Read the model definition and answer for the solid it produces. Units are mm, in the model's axes. A direction names the side the tool comes from. Give positions to 0.01 mm unless a question says otherwise; leave off trailing zeros. Order: outer loops, then holes, each group sorted by start corner. A loop starts at its lowest first (then second) coordinate and runs counter-clockwise, first axis right, second up. Notation, with made-up numbers: (72, 81) - (104, 81) arc R19 ccw to (104, 111) - close; hole circle Ø7 at (-25, 81.5). An arc over 180 degrees is marked (long way). Use a Markdown table: item, result. Add a question column.
1. Which of the six approach directions +Z, -Z, +X, -X, +Y, -Y give full straight-line access (tool end or side, diameter ignored) to faces 5 (the flat face through (11.112, 20, 1)), 6 (the cylindrical face through (0.22, 9.65, 1.48))?
2. A cutting plane is placed at C-C on y = 61.5. Determine the outline of the cut face in (x, z), and give its area (3 significant figures).
3. A cutting plane is placed at B-B on z = 2.3. Determine the outline of the cut face in (x, y) (1 decimal), and give its area (3 significant figures).
4. Flat-ended cylindrical pins translate along their axes: P1, Ø5.5, axis at x = 0, y = -7.94, coming from the -Z side; P2, Ø1.5, axis at y = 11, z = 2, coming from the +X side. Find the tip coordinate at first contact, or state that the pin passes through.
5. A cutting plane is placed at A-A on x = 0. Determine the outline of the cut face in (y, z), and give its area (3 significant figures).
6. A cutting plane is placed at D-D on x = 17.5. Determine the outline of the cut face in (y, z), and give its area (3 significant figures).
7. For a pull along X with two mould halves and no side action, classify faces 1 (the flat face through (4, 46, 3)), 2 (the cylindrical face through (-0.22, -11.11, 1.48)), 3 (the cylindrical face through (0.225, -6.225, 1.479)), 4 (the cylindrical face through (-6.212, 0.076, 1.479)) as released by +X, released by -X, zero draft, split by the parting line, or undercut.
8. Consider L1, parallel to Y at x = 21.5, z = 2.4; L2, parallel to X at y = 24, z = 0.85; L3, parallel to X at y = 88.5, z = 2. Determine where each line is inside the solid, lowest interval first.
```python
from build123d import *

# Parameters (mm, degrees)
BOSS_EXTRU_3_DEPTH   = 3
D_GAGEMENT_51_D      = 3.4544
D_GAGEMENT_M71_D     = 7.6
D_GAGEMENT_M71_DEPTH = 7.01
D_GAGEMENT_M71_TIP   = 2.283270352


with BuildPart() as part:
    # Esquisse1 → Boss.-Extru.3 (new body)
    with BuildSketch(Plane.XY):
        with BuildLine():
            Line((11.1125, 0), (11.1125, 40))
            ThreePointArc((11.1125, 40), (15.168988239, 68.192952149), (27.009351017, 94.098616722))
            ThreePointArc((27.009351017, 94.098616722), (25.537478416, 100.990911223), (18.635346271, 99.565883395))
            ThreePointArc((18.635346271, 99.565883395), (-3.639418742, 51.966145876), (-11.112370677, -0.053611501))
            ThreePointArc((-11.112370677, -0.053611501), (0.026805829, -11.112467669), (11.1125, 0))
        make_face()
    extrude(amount=BOSS_EXTRU_3_DEPTH)

    # Dégagement #51 (through all)
    with Locations(Plane.XY.offset(3)):
        with Locations((-7.9375, 0), (0, 7.9375), (7.9375, 0), (0, -7.9375)):
            Hole(D_GAGEMENT_51_D / 2)

    # Dégagement M71
    with Locations(Plane.XY.offset(3)):
        with Locations((0, 0)):
            Hole(D_GAGEMENT_M71_D / 2, depth=D_GAGEMENT_M71_DEPTH)
            with Locations((0, 0, -(D_GAGEMENT_M71_DEPTH + D_GAGEMENT_M71_TIP / 2))):  # 118° drill point
                Cone(0, D_GAGEMENT_M71_D / 2, D_GAGEMENT_M71_TIP, mode=Mode.SUBTRACT)


solid = part.part
```
Output values:
| question | item | result |
|---|---|---|
| 1 | face 5 | +Z, -Z, +X, -Y |
| 1 | face 6 | +Z, -Z |
| 2 | outline | (-0.5, 0) - (13.45, 0) - (13.45, 3) - (-0.5, 3) - close |
| 2 | area | 41.8 mm² |
| 3 | outline | (-11.1, -0.1) arc R11.1 ccw to (11.1, 0) - (11.1, 40) arc R100 cw to (27, 94.1) arc R5 ccw to (18.6, 99.6) arc R178.8 ccw to start; hole circle Ø3.5 at (-7.9, 0); hole circle Ø7.6 at (0, 0); hole circle Ø3.5 at (0, -7.9); hole circle Ø3.5 at (0, 7.9); hole circle Ø3.5 at (7.9, 0) |
| 3 | area | 1,760 mm² |
| 4 | P1 | z = 0 |
| 4 | P2 | x = 11.11 |
| 5 | outline | (-11.11, 0) - (-9.66, 0) - (-9.66, 3) - (-11.11, 3) - close; (-6.21, 0) - (-3.8, 0) - (-3.8, 3) - (-6.21, 3) - close; (3.8, 0) - (6.21, 0) - (6.21, 3) - (3.8, 3) - close; (9.66, 0) - (62.86, 0) - (62.86, 3) - (9.66, 3) - close |
| 5 | area | 178 mm² |
| 6 | outline | (75.17, 0) - (97.83, 0) - (97.83, 3) - (75.17, 3) - close |
| 6 | area | 68.0 mm² |
| 7 | face 1 | zero draft |
| 7 | face 2 | split by the parting line |
| 7 | face 3 | undercut |
| 7 | face 4 | undercut |
| 8 | L1 | 84.38 to 101.63 |
| 8 | L2 | -9.6 to 11.11 |
| 8 | L3 | 11.87 to 23.66 |
